Read the model definition and answer for the solid it produces. Units are mm, in the model's axes. Round coordinates to 2 decimals unless told otherwise and drop trailing zeros. Order: outer loops, then holes, each group sorted by start corner. A loop starts at its lowest first (then second) coordinate and runs counter-clockwise, first axis right, second up. Notation, with made-up numbers: (5.5, 48) -> (53.5, 48) arc R27 ccw to (53.5, 67) -> close; hole circle Ø9 at (-29.5, 75). An arc over 180 degrees is marked (long way). Use a Markdown table: item, result. Add a question column.
1. Section B-B, the plane z = 12.7 is taken. Give the vertices of the cut face in (x, y).
2. Consider L1, parallel to X at y = -23.25, z = 14.5; L2, parallel to Z at x = -127, y = -7.75; L3, parallel to X at y = -14, z = 9.75. Determine where each line is inside the solid, lowest interval first. Write a range as [from, to].
3. Section A-A, the plane x = 127 is taken. Give the vertices of the cut face in (y, z), then the cut area to 3 significant figures.
4. The mould has two halves that part along X. Classify faces 1 (the face through (190.5, -13, 13)), 2 (the face through (3.414, -12.878, 18.054)), 3 (the face through (-3, -25.4, 19)): +X half, -X half, draft (parallel to the pull), parting line (faces both ways), or undercut.
5. Given pin 1 (11.5 mm diameter, centred on x = -127, z = 12.7, fed in from +Y), flat-ended and moving along its own axis, determine where the tip first touches the part or whether it passes through.
6. Section C-C, the plane y = -20.25 is taken. Give the vertices of the cut face in (x, z), then the cut area to 3 significant figures.
```python
from build123d import *

# Parameters (mm, degrees)
F1_DEPTH = 25.4
F2_R     = 6.35
F3_DEPTH = 50.8
F4_SIZE  = 5.08
F5_SIZE  = 5.08


with BuildPart() as f1:
    # F0 (on Front) → F1 (new body)
    with BuildSketch(Plane.XZ):
        Polygon((-190.5, 0), (0, 0), (190.5, 0), (190.5, 25.4), (-190.5, 25.4), align=None)
    extrude(amount=F1_DEPTH)

    # F2 (on face) → F3 (cut)
    with BuildSketch(Plane.XZ.offset(25.4)):
        with Locations((-127, 12.7)):
            Circle(F2_R)
        with Locations((0, 12.7)):
            Circle(F2_R)
        with Locations((127, 12.7)):
            Circle(F2_R)
    extrude(amount=-F3_DEPTH, mode=Mode.SUBTRACT)

    # F4
    f4_edges = [f1.edges().sort_by_distance(p)[0] for p in [
        (-190.5, -12.7, 25.4),
    ]]
    chamfer(f4_edges, length=F4_SIZE)

    # F5
    f5_edges = [f1.edges().sort_by_distance(p)[0] for p in [
        (-190.5, -12.7, 0),
        (190.5, -12.7, 25.4),
        (190.5, -12.7, 0),
    ]]
    chamfer(f5_edges, length=F5_SIZE)


solid = f1.part
```
Verdict:
| question | item | result |
|---|---|---|
| 1 | outline | (-190.5, -25.4) -> (-133.35, -25.4) -> (-133.35, 0) -> (-190.5, 0) -> close; (-120.65, -25.4) -> (-6.35, -25.4) -> (-6.35, 0) -> (-120.65, 0) -> close; (6.35, -25.4) -> (120.65, -25.4) -> (120.65, 0) -> (6.35, 0) -> close; (133.35, -25.4) -> (190.5, -25.4) -> (190.5, 0) -> (133.35, 0) -> close |
| 2 | L1 | x = [-190.5, -133.09], [-120.91, -6.09], [6.09, 120.91], [133.09, 190.5] |
| 2 | L2 | z = [0, 6.35], [19.05, 25.4] |
| 2 | L3 | x = [-190.5, -132.62], [-121.38, -5.62], [5.62, 121.38], [132.62, 190.5] |
| 3 | outline | (-25.4, 0) -> (0, 0) -> (0, 6.35) -> (-25.4, 6.35) -> close; (-25.4, 19.05) -> (0, 19.05) -> (0, 25.4) -> (-25.4, 25.4) -> close |
| 3 | area | 323 mm2 |
| 4 | face 1 | +X half |
| 4 | face 2 | undercut |
| 4 | face 3 | draft |
| 5 | pin 1 | passes through |
| 6 | outline | (-190.5, 5.08) -> (-185.42, 0) -> (185.42, 0) -> (190.5, 5.08) -> (190.5, 20.32) -> (185.42, 25.4) -> (-185.42, 25.4) -> (-190.5, 20.32) -> close; hole circle Ø12.7 at (-127, 12.7); hole circle Ø12.7 at (0, 12.7); hole circle Ø12.7 at (127, 12.7) |
| 6 | area | 9,250 mm2 |
